```python
from build123d import *

# Parameters (mm, degrees)
SKETCH1_R           = 11.049
BOSS_EXTRUDE1_DEPTH = 452.12
SKETCH2_R           = 4
BOSS_EXTRUDE2_DEPTH = 8.382
CHAMFER1_SIZE       = 0.762
FILLET1_R           = 1.905
SKETCH3_R           = 4.953
CUT_EXTRUDE1_DEPTH  = 431.8


with BuildPart() as part:
    # Sketch1 → Boss-Extrude1 (new body)
    with BuildSketch(Plane(origin=(0, 0, 0), x_dir=(1, 0, 0), z_dir=(0, 1, 0))):
        with Locations(Location((0, 0, 0), (0, 0, 90))):
            Circle(SKETCH1_R)
    extrude(amount=BOSS_EXTRUDE1_DEPTH)

    # Sketch2 → Boss-Extrude2 (add)
    with BuildSketch(Plane(origin=(0, 452.12, 0), x_dir=(1, 0, 0), z_dir=(0, 1, 0))):
        with Locations(Location((0, 0, 0), (0, 0, 270))):
            Circle(SKETCH2_R)
    extrude(amount=BOSS_EXTRUDE2_DEPTH)

    # Chamfer1
    chamfer1_edges = [part.edges().sort_by_distance(p)[0] for p in [
        (0, 460.502, -4),
    ]]
    chamfer(chamfer1_edges, length=CHAMFER1_SIZE)

    # Fillet1
    fillet1_edges = [part.edges().sort_by_distance(p)[0] for p in [
        (0, 0, 11.049),
        (0, 452.12, 11.049),
    ]]
    fillet(fillet1_edges, radius=FILLET1_R)

    # Sketch3 → Cut-Extrude1 (cut)
    with BuildSketch(Plane.XZ):
        with Locations(Location((0, 0, 0), (0, 0, 270))):
            Circle(SKETCH3_R)
    extrude(amount=-CUT_EXTRUDE1_DEPTH, mode=Mode.SUBTRACT)


solid = part.part
```
Read the model definition and answer for the solid it produces. Units are mm, in the model's axes. A direction names the side the tool comes from. Coordinates: 2 decimals unless noted, no trailing zeros. Loops run counter-clockwise (first coordinate to the right, second up) from the corner with the lowest first, then second, coordinate; pieces in that order, holes last. Notation, with made-up numbers: (-4, 81) -> (52, 81) arc R25 cw to (52, 116) -> close; hole circle Ø9 at (63.25, 1.25). An arc over 180 degrees is marked (long way). Return JSON: item names as keys, results as strings.
Item 1: Find section A-A (y = 132.5). Determine the outline of the cut face in (x, z), plus the area to 3 significant figures.
Answers:
{"outline": "circle Ø22.1 at (0, 0); hole circle Ø9.91 at (0, 0)", "area": "306 mm2"}
Item 2: Find the intervals of material crossed by probe 1 along X at (y, z) = (331, 0); probe 2 along Z at (x, y) = (-0.5, 88.5); probe 3 along X at (y, z) = (221, -0.75), in increasing order.
Answers:
{"probe 1": "x = -11.05 to -4.95, 4.95 to 11.05", "probe 2": "z = -11.04 to -4.93, 4.93 to 11.04", "probe 3": "x = -11.02 to -4.9, 4.9 to 11.02"}
Item 3: For faces 4 (the flat face through (0, 431.8, 0)), 5 (the cylindrical face through (-7.47, 222.92, 8.14)), determine the directions among +Z, -Z, +X, -X, +Y, -Y from which every point of the face is accessible in a straight line to the end or side of a thin tool.
Answers:
{"face 4": "-Y", "face 5": "+Y, -Y"}
Item 4: Flat-ended cylindrical pins translate along their axes: P1, Ø6, axis at y = 137.5, z = -5, coming from the +X side; P2, Ø3, axis at x = -1, z = -1.5, coming from the -Y side; P3, Ø1.5, axis at x = 5.5, z = -2, coming from the +Y side. Find the tip coordinate at first contact, or state that the pin passes through.
Answers:
{"P1": "stops at x = 10.87", "P2": "stops at y = 431.8", "P3": "stops at y = 452.12"}
Item 5: For a pull along Z with two mould halves and no side action, classify faces 1 (the cylindrical face through (1.488, 212.877, -4.724)), 2 (the cylindrical face through (-3.905, 455.877, -0.867)), 3 (the flat face through (2, 452.12, -4)) as +Z half, -Z half, draft (parallel to the pull), parting line (faces both ways), or undercut.
Answers:
{"face 1": "undercut", "face 2": "parting line", "face 3": "draft"}
